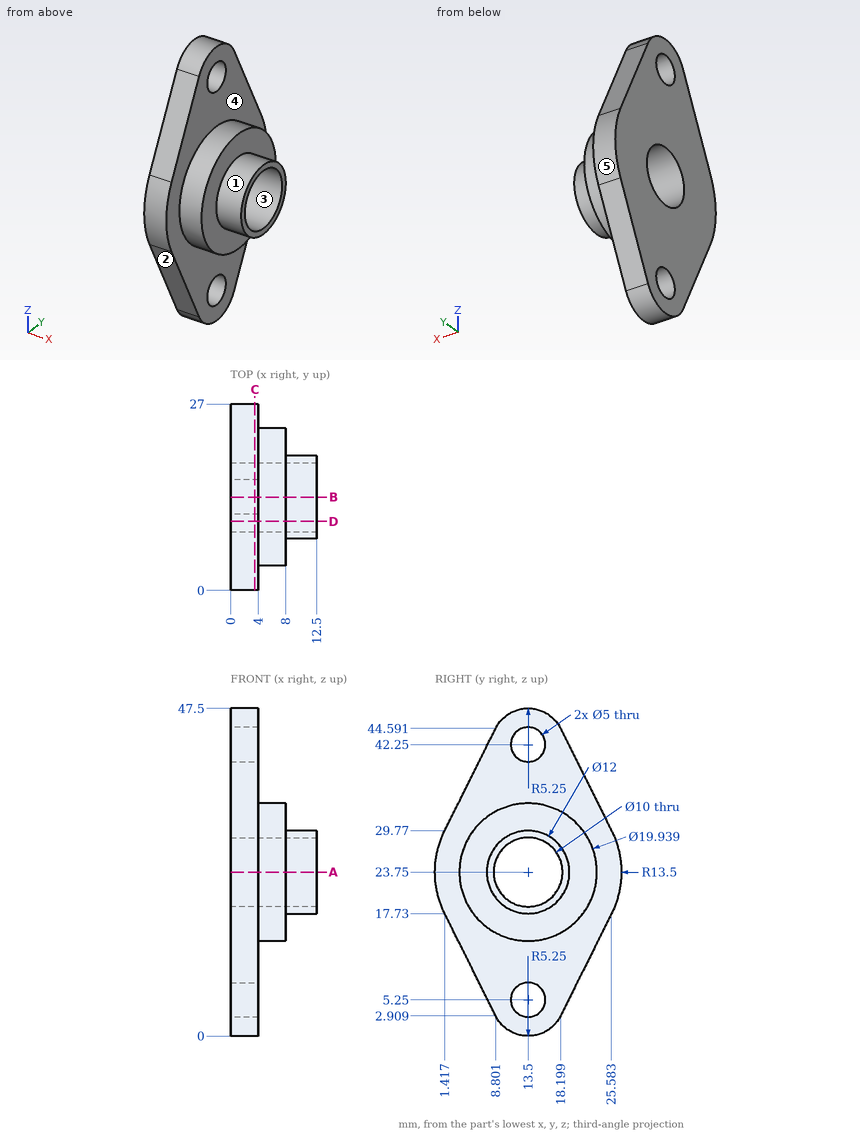
Design review of the part shown in the three views and the two pictorial views. Dimensions are in mm from the part's minimum x, y and z. A direction names the side the tool comes from. Give positions to 0.01 mm unless a question says otherwise; leave off trailing zeros. Write each loop counter-clockwise with the first axis right and the second up, starting at its lowest first coordinate (ties: lowest second). Pieces come first, ordered by that corner, then holes. Notation, with made-up numbers: M 47,79.25 L 89,79.25 A22 ccw 89,117.25 Z; hole C 39.25,-19.75 d11. An arc over 180 degrees is marked long. One line per question, with ' | ' between items. Start each with the question number.
Item 1: Wall thickness on line 1 (Y direction, x = 8.75, z = 23.75); line 2 (X direction, y = 11, z = 12.5); line 3 (X direction, y = 11, z = 32): over which ranges is each line inside the solid? List them lowest first. Write a range as from..to.
Item 2: For the marked faces 4 and 5, list the 3-axis set-ups (+Z, -Z, +X, -X, +Y, -Y) from which the entire face can be reached by the end or side of a thin tool; tool diameter is ignored.
Item 3: We need section C-C on x = 3.5. Write out the cut boundary in (y, z).
Item 4: For pin 1 (4 mm diameter, centred on x = 3, z = 15, fed in from +Y); pin 2 (3 mm diameter, centred on x = 6.5, z = 34, fed in from +Y); pin 3 (3 mm diameter, centred on x = 2.5, y = 17.5, fed in from -Z), all flat-tipped, find the tip position at first contact; note any pin that passes through.
Item 5: We need section A-A on z = 23.75. Write out the cut boundary in (x, y).
Item 6: We need section D-D on y = 10. Write out the cut boundary in (x, z) (1 decimal).
Item 7: Draft analysis for pull direction Y (two halves, no side actions). For the marked faces 1, 2 and 3, state which applies: released by +Y, released by -Y, zero draft, split by the parting line, or undercut.
Item 8: We need section B-B on y = 13.5. Write out the cut boundary in (x, z), plus the area to 3 significant figures.
Results found:
1) line 1: y = 7.5..8.5, 18.5..19.5 | line 2: x = 0..4 | line 3: x = 0..8
2) face 4: +X | face 5: +X, -X, +Y
3) outline: M 1.42,17.73 L 8.8,2.91 A5.25 ccw 18.2,2.91 L 25.58,17.73 A13.5 ccw 25.58,29.77 L 18.2,44.59 A5.25 ccw 8.8,44.59 L 1.42,29.77 A13.5 ccw Z; hole C 13.5,23.75 d10; hole C 13.5,5.25 d5; hole C 13.5,42.25 d5
4) pin 1: stops at y = 25.22 | pin 2: stops at y = 18.28 | pin 3: stops at z = 0.63
5) outline: M 0,0 L 4,0 L 4,3.53 L 8,3.53 L 8,7.5 L 12.5,7.5 L 12.5,8.5 L 0,8.5 Z; M 0,18.5 L 12.5,18.5 L 12.5,19.5 L 8,19.5 L 8,23.47 L 4,23.47 L 4,27 L 0,27 Z
6) outline: M 0,1.3 L 4,1.3 L 4,14.4 L 8,14.4 L 8,18.9 L 12.5,18.9 L 12.5,20.2 L 0,20.2 Z; M 0,27.3 L 12.5,27.3 L 12.5,28.6 L 8,28.6 L 8,33.1 L 4,33.1 L 4,46.2 L 0,46.2 Z
7) face 1: split by the parting line | face 2: released by -Y | face 3: undercut
8) outline: M 0,0 L 4,0 L 4,2.75 L 0,2.75 Z; M 0,7.75 L 4,7.75 L 4,13.78 L 8,13.78 L 8,17.75 L 12.5,17.75 L 12.5,18.75 L 0,18.75 Z; M 0,28.75 L 12.5,28.75 L 12.5,29.75 L 8,29.75 L 8,33.72 L 4,33.72 L 4,39.75 L 0,39.75 Z; M 0,44.75 L 4,44.75 L 4,47.5 L 0,47.5 Z | area: 159 mm2
